Autodesk Fusion 360 part; units mm, degrees
sketch "Sketch3" plane through (0, 0, 0) normal (0, 0, 1) x (1, 0, 0)
  line L0 (50, -20) -> (-50, -20)
  line L1 (-50, -20) -> (-50, 20)
  line L2 (-50, 20) -> (50, 20)
  line L3 (50, 20) -> (50, -20)
  line L4 (50, -20) -> (-50, 20) construction
  line L5 (-50, -20) -> (50, 20) construction
  line L6 (35, -4) -> (-35, -4)
  line L7 (-35, -4) -> (-35, 4)
  line L8 (-35, 4) -> (35, 4)
  line L9 (35, 4) -> (35, -4)
  line L10 (35, -4) -> (-35, 4) construction
  line L11 (-35, -4) -> (35, 4) construction
  line L12 (50, 20) -> (58, 20)
  line L13 (58, 20) -> (58, -20)
  line L14 (58, -20) -> (50, -20)
  line L15 (50, -20) -> (50, 20)
  circle A0 centre (-35, 0) radius 4
  circle A1 centre (35, 0) radius 4
  dimension "d9" = 100
  dimension "d10" = 40
  dimension "d11" = 70
  dimension "d12" = 8
  dimension "d14" = 8
  dimension "d15" = 40
  dimension "d16" = 8
  dimension "d17" = 8
extrude "Extrude1" add sketch "Sketch3" along normal blind 11.3 contours L0 L1 L2 L3 L15
extrude "Extrude2" add sketch "Sketch3" along normal blind 6.3 contours L3 L12 L13 L14 L15
fillet "Fillet1" radius 5 4 edges at (-50, -20, 5.65) (-50, 20, 5.65) (58, 20, 3.15) (58, -20, 3.15)
equation "thickness = 11.3 mm"
equation "largeur = 40 mm"
equation "longueurTotal = 100 mm"
equation "diametre = 8 mm"
equation "epaulement = thickness - 5 mm"
equation "longueurRainure = longueurTotal - 30 mm"
equation "largeurRainure = 8 mm"
equation "d9 = longueurTotal"
equation "d10 = largeur"
equation "d11 = longueurRainure"
equation "d12 = largeurRainure"
equation "largeurEpaulement = 8 mm"
equation "d14 = largeurEpaulement"
equation "d15 = largeur"
equation "d16 = diametre"
equation "d17 = diametre"
equation "d18 = thickness"
equation "d20 = epaulement"
Build history of the part. All positions in model axes, mm. A direction names the side the tool comes from. Give positions to 0.01 mm unless a question says otherwise; leave off trailing zeros. Loops run counter-clockwise (first coordinate to the right, second up) from the corner with the lowest first, then second, coordinate; pieces in that order, holes last. Notation, with made-up numbers: (69.25, -19) - (82.25, -19) arc R16 cw to (82.25, -4) - close; hole circle Ø5 at (-11.75, -30.75). An arc over 180 degrees is marked (long way). Write item = value, one per line. Start each with the question number.
1) Tool access for faces 1 (the cylindrical face through (-39, 0, 6)), 2 (the flat face through (54, 0, 6.3)), 3 (the cylindrical face through (-49, -18, 6)): list every direction of +Z, -Z, +X, -X, +Y, -Y with a clear straight run to the whole face (end or side of a thin tool).
2) Band-saw the part on A-A on x = 3.5. Give the cut face in (y, z).
3) Band-saw the part on C-C on y = -0.5. Give the cut face in (x, z).
4) Band-saw the part on B-B on z = 9. Give the cut face in (x, y).
5) Drop flat-ended pins along their axis: pin 1 Ø4 at (x, y) = (55.5, -8) entering from +Z; pin 2 Ø1.5 at (y, z) = (1, 7.5) entering from +X. Give the stop position or say it passes through.
6) Band-saw the part on D-D on y = 8. Give the cut face in (x, z), plus the area to 3 significant figures.
7) Probe probe 1 along Y at (x, z) = (-5, 7.75); probe 2 along X at (y, z) = (-0.5, 4.5); probe 3 along Y at (x, z) = (-36, 5.5). List the from-to ranges inside material, lowest first. Write a range as from..to.
8) Pull direction X, two halves, no side cores. Call faces 4 (the flat face through (3.2, -4.2, 0)), 5 (the flat face through (50, 0, 9)), 6 (the flat face through (0, 4, 6)): +X half, -X half, draft (parallel to the pull), parting line (faces both ways), or undercut.
Final values:
q1.face_1 = +Z, -Z
q1.face_2 = +Z, +X, +Y, -Y
q1.face_3 = +Z, -Z, -X, -Y
q2.outline = (-20, 0) - (-4, 0) - (-4, 11.3) - (-20, 11.3) - close; (4, 0) - (20, 0) - (20, 11.3) - (4, 11.3) - close
q3.outline = (-50, 0) - (-38.97, 0) - (-38.97, 11.3) - (-50, 11.3) - close; (38.97, 0) - (58, 0) - (58, 6.3) - (50, 6.3) - (50, 11.3) - (38.97, 11.3) - close
q4.outline = (-50, -15) arc R5 ccw to (-45, -20) - (50, -20) - (50, 20) - (-45, 20) arc R5 ccw to (-50, 15) - close; hole (-35, -4) - (35, -4) arc R4 ccw to (35, 4) - (-35, 4) arc R4 ccw to start
q5.pin_1 = 6.3
q5.pin_2 = 50
q6.outline = (-50, 0) - (58, 0) - (58, 6.3) - (50, 6.3) - (50, 11.3) - (-50, 11.3) - close
q6.area = 1,180 mm²
q7.probe_1 = -20..-4, 4..20
q7.probe_2 = -50..-38.97, 38.97..58
q7.probe_3 = -20..-3.87, 3.87..20
q8.face_4 = draft
q8.face_5 = +X half
q8.face_6 = undercut
